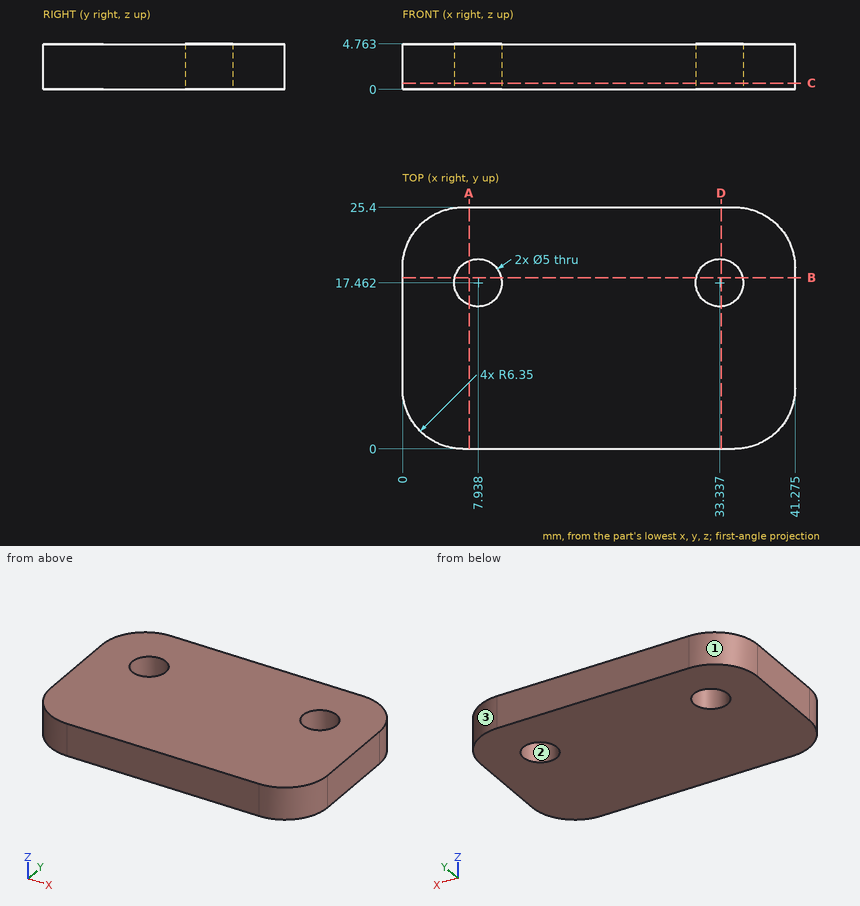
Could you check a few things on this drawing? It's one solid part, dimensions in mm from its lowest x, y, z. Give positions to 0.01 mm unless a question says otherwise; leave off trailing zeros. Order: outer loops, then holes, each group sorted by start corner. A loop starts at its lowest first (then second) coordinate and runs counter-clockwise, first axis right, second up.
1. Suppose I cut it at A-A (x = 7). Write out the boundary of the cut face in (y, z) (1 decimal).
Answers below:
outline: (0, 0) - (15.1, 0) - (15.1, 4.8) - (0, 4.8) - close; (19.8, 0) - (25.4, 0) - (25.4, 4.8) - (19.8, 4.8) - close
2. I need wall thicknesses on L1, parallel to Y at x = 6.5, z = 4.3 (1 decimal); L2, parallel to X at y = 15.5, z = 4.25 (1 decimal); L3, parallel to Y at x = 33, z = 0.6 (1 decimal). Which ranges of each line are inside material? Lowest first, please.
Answers below:
L1: y = 0 to 15.4, 19.5 to 25.4
L2: x = 0 to 6.4, 9.5 to 31.8, 34.9 to 41.3
L3: y = 0 to 15, 19.9 to 25.4
3. Suppose I cut it at B-B (y = 18). Write out the boundary of the cut face in (x, z) (1 decimal).
Answers below:
outline: (0, 0) - (5.5, 0) - (5.5, 4.8) - (0, 4.8) - close; (10.4, 0) - (30.9, 0) - (30.9, 4.8) - (10.4, 4.8) - close; (35.8, 0) - (41.3, 0) - (41.3, 4.8) - (35.8, 4.8) - close
4. Suppose I cut it at C-C (z = 0.65). State how many separate pieces and enclosed holes the cut face has.
Answers below:
separate pieces: 1
enclosed holes: 2
5. For pin 1 (4 mm diameter, centred on x = 33.34, y = 17.46, fed in from +Z), with a flat end and sliding along its axis, tell me the tip position at first contact or that it passes through.
Answers below:
pin 1: passes through
6. Suppose I cut it at D-D (x = 33.5). Write out the boundary of the cut face in (y, z).
Answers below:
outline: (0, 0) - (14.97, 0) - (14.97, 4.76) - (0, 4.76) - close; (19.96, 0) - (25.4, 0) - (25.4, 4.76) - (19.96, 4.76) - close
7. Thinking about a two-plate mould opening in X: for the marked faces 1, 2 and 3, which applies, +X half, -X half, draft (parallel to the pull), parting line (faces both ways), or undercut?
Answers below:
face 1: -X half
face 2: undercut
face 3: +X half
